Job drawing, mm, ordinate dimensions from the low corner. One solid piece. A direction names the side the tool comes from. Round coordinates to 2 decimals unless told otherwise and drop trailing zeros. Order: outer loops, then holes, each group sorted by start corner. A loop starts at its lowest first (then second) coordinate and runs counter-clockwise, first axis right, second up. Notation, with made-up numbers: (16.25, 7) -> (68.25, 7) arc R25 ccw to (68.25, 21) -> close; hole circle Ø6 at (66.25, 51.5). An arc over 180 degrees is marked (long way). Return JSON: item names as keys, results as strings. Group by question number.
Q1. Cut at B-B (x = 45). Write the cut outline in (y, z), then the cut area to 3 significant figures.
Q2. Cut at D-D (z = 20.5). Write the cut outline in (x, y) (3 decimals), then the cut area to 3 significant figures.
Q3. Flat gauge pins, fed straight in: pin 1 (4 mm diameter, centred on y = 41, z = 14.5, fed in from +X); pin 2 (1.5 mm diameter, centred on x = 23.5, y = 25, fed in from -Z); pin 3 (4 mm diameter, centred on x = 14, z = 19, fed in from -Y). Where does each tip first touch, or does it go through?
Q4. Cut at C-C (x = 6.5). Write the cut outline in (y, z), then the cut area to 3 significant figures.
Q5. Probe line 1 along Y through (x, z) = (45, 12); line 2 along X through (y, z) = (23, 22); line 3 along X through (y, z) = (23, 16). List the from-to ranges inside material, lowest first.
Q6. Which spindle directions (+Z, -Z, +X, -X, +Y, -Y) get a long thin tool onto all of the face, cutting with end or side? Do the marked faces 1, 2, 3, 4 and 5. Say none if no direction does.
Q7. Cut at A-A (z = 15.5). Write the cut outline in (x, y), then the cut area to 3 significant figures.
Q8. Mould opens along Y. For the marked faces 6, 7, 8 and 9 say: +Y half, -Y half, draft (parallel to the pull), parting line (faces both ways), or undercut.
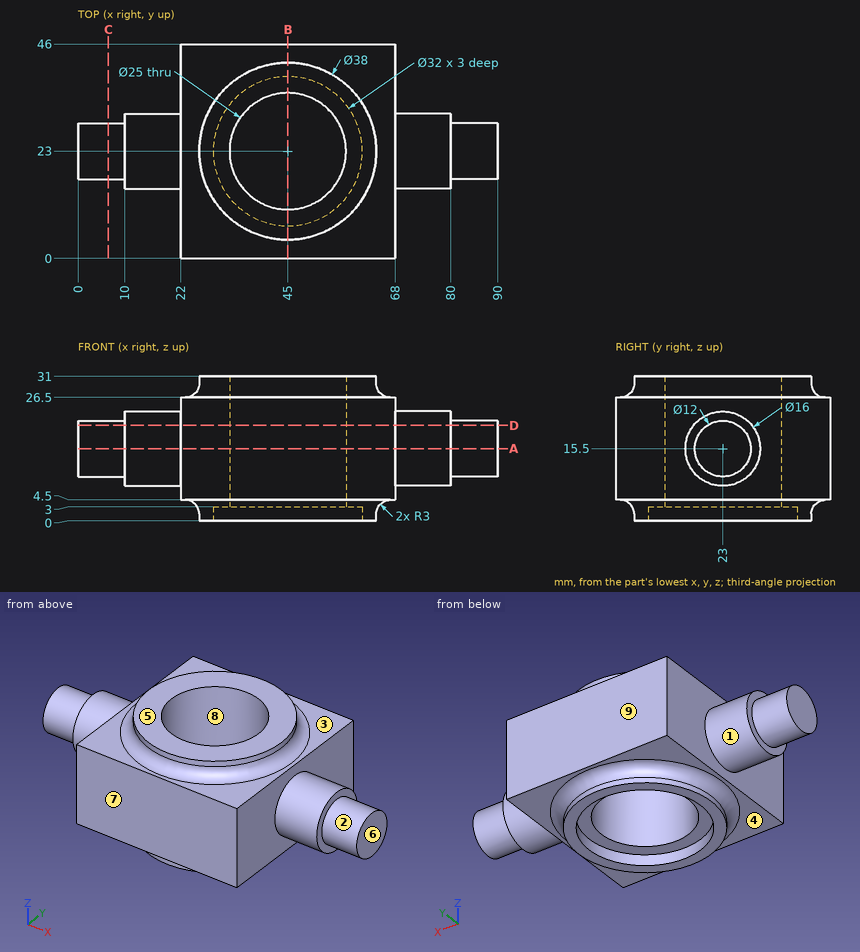
Solution:
{
 "1": {"outline": "(0, 4.5) -> (1, 4.5) arc R3 cw to (4, 1.5) -> (4, 0) -> (7, 0) -> (7, 3) -> (10.5, 3) -> (10.5, 31) -> (4, 31) -> (4, 29.5) arc R3 cw to (1, 26.5) -> (0, 26.5) -> close; (35.5, 3) -> (39, 3) -> (39, 0) -> (42, 0) -> (42, 1.5) arc R3 cw to (45, 4.5) -> (46, 4.5) -> (46, 26.5) -> (45, 26.5) arc R3 cw to (42, 29.5) -> (42, 31) -> (35.5, 31) -> close", "area": "566 mm²"},
 "2": {"outline": "(0, 19.683) -> (10, 19.683) -> (10, 16.755) -> (22, 16.755) -> (22, 0) -> (68, 0) -> (68, 16.755) -> (80, 16.755) -> (80, 19.683) -> (90, 19.683) -> (90, 26.317) -> (80, 26.317) -> (80, 29.245) -> (68, 29.245) -> (68, 46) -> (22, 46) -> (22, 29.245) -> (10, 29.245) -> (10, 26.317) -> (0, 26.317) -> close; hole circle Ø25 at (45, 23)", "area": "2,060 mm²"},
 "3": {"pin 1": "stops at x = 68", "pin 2": "stops at z = 4.27", "pin 3": "stops at y = 15.14"},
 "4": {"outline": "circle Ø12 at (23, 15.5)", "area": "113 mm²"},
 "5": {"line 1": "y = 0 to 10.5, 35.5 to 46", "line 2": "x = 10 to 32.5, 57.5 to 80", "line 3": "x = 0 to 32.5, 57.5 to 90"},
 "6": {"face 1": "-X", "face 2": "+X", "face 3": "+Z", "face 4": "-Z", "face 5": "+Z, +X, -X, +Y, -Y"},
 "7": {"outline": "(0, 17) -> (10, 17) -> (10, 15) -> (22, 15) -> (22, 0) -> (68, 0) -> (68, 15) -> (80, 15) -> (80, 17) -> (90, 17) -> (90, 29) -> (80, 29) -> (80, 31) -> (68, 31) -> (68, 46) -> (22, 46) -> (22, 31) -> (10, 31) -> (10, 29) -> (0, 29) -> close; hole circle Ø25 at (45, 23)", "area": "2,250 mm²"},
 "8": {"face 6": "draft", "face 7": "-Y half", "face 8": "undercut", "face 9": "+Y half"}
}
